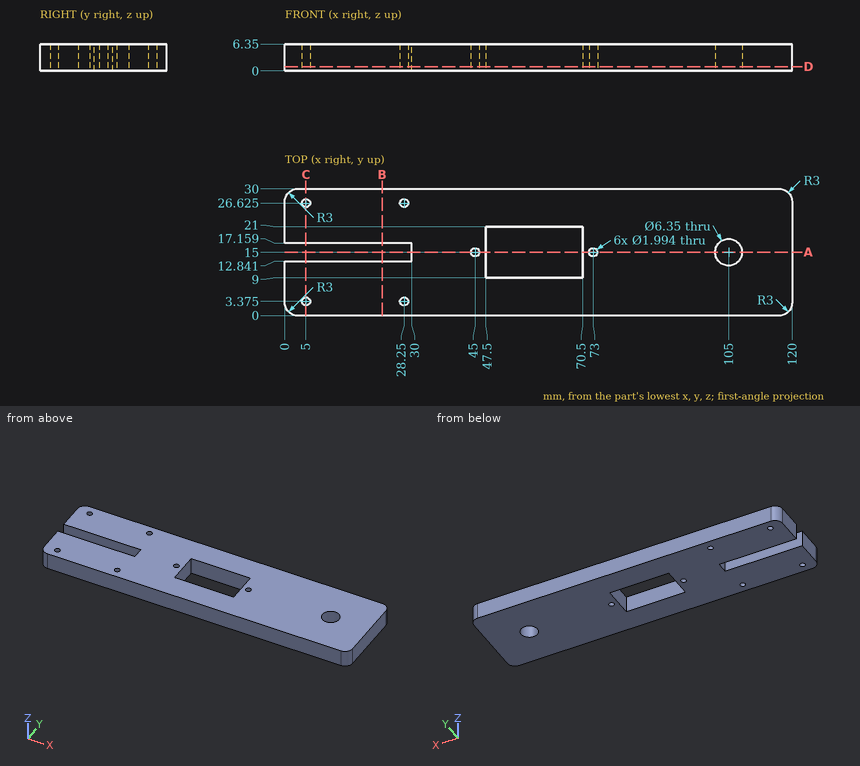
Input: dimensioned drawing with shaded views. Units: mm. Origin: part minimum x, y, z. Coordinates: 2 decimals unless noted, no trailing zeros. Loops run counter-clockwise (first coordinate to the right, second up) from the corner with the lowest first, then second, coordinate; pieces in that order, holes last. Notation, with made-up numbers: (-27, -11) -> (23, -11) arc R14 ccw to (23, 1) -> close; hole circle Ø4 at (58.25, 29). An arc over 180 degrees is marked (long way). Use a Markdown table: item, result. Add a question column.
(1) Line query: line 1 along Y through (x, z) = (5, 3); line 2 along Y through (x, z) = (23, 0.5); line 3 along X through (y, z) = (20.25, 0.5). Output: solid intervals per line, ascending.
(2) Section query D-D, the plane z = 1. State how many separate pieces and enclosed holes the cut face has, plus the area to 3 significant figures.
(3) Section query A-A, the plane y = 15. Return loops of the section in (x, z) (3 decimals), plus the area to 3 significant figures.
(4) Section query C-C, the plane x = 5. Return loops of the section in (y, z), plus the area to 3 significant figures.
(5) Section query B-B, the plane x = 23. Return loops of the section in (y, z), plus the area to 3 significant figures.
Answer:
| question | item | result |
|---|---|---|
| 1 | line 1 | y = 0 to 2.38, 4.37 to 12.84, 17.16 to 25.63, 27.62 to 30 |
| 1 | line 2 | y = 0 to 12.84, 17.16 to 30 |
| 1 | line 3 | x = 0 to 47.5, 70.5 to 120 |
| 2 | separate pieces | 1 |
| 2 | enclosed holes | 8 |
| 2 | area | 3,140 mm^2 |
| 3 | outline | (30, 0) -> (44.003, 0) -> (44.003, 6.35) -> (30, 6.35) -> close; (45.997, 0) -> (47.5, 0) -> (47.5, 6.35) -> (45.997, 6.35) -> close; (70.5, 0) -> (72.003, 0) -> (72.003, 6.35) -> (70.5, 6.35) -> close; (73.997, 0) -> (101.825, 0) -> (101.825, 6.35) -> (73.997, 6.35) -> close; (108.175, 0) -> (120, 0) -> (120, 6.35) -> (108.175, 6.35) -> close |
| 3 | area | 360 mm^2 |
| 4 | outline | (0, 0) -> (2.38, 0) -> (2.38, 6.35) -> (0, 6.35) -> close; (4.37, 0) -> (12.84, 0) -> (12.84, 6.35) -> (4.37, 6.35) -> close; (17.16, 0) -> (25.63, 0) -> (25.63, 6.35) -> (17.16, 6.35) -> close; (27.62, 0) -> (30, 0) -> (30, 6.35) -> (27.62, 6.35) -> close |
| 4 | area | 138 mm^2 |
| 5 | outline | (0, 0) -> (12.84, 0) -> (12.84, 6.35) -> (0, 6.35) -> close; (17.16, 0) -> (30, 0) -> (30, 6.35) -> (17.16, 6.35) -> close |
| 5 | area | 163 mm^2 |
